Design review of the part shown in the three views and the two pictorial views. Dimensions are in mm from the part's minimum x, y and z. Round coordinates to 2 decimals unless told otherwise and drop trailing zeros. Loops run counter-clockwise (first coordinate to the right, second up) from the corner with the lowest first, then second, coordinate; pieces in that order, holes last. Notation, with made-up numbers: M 86.5,63 L 145.5,63 A23 cw 145.5,98 Z; hole C -7.5,-12 d7. An arc over 180 degrees is marked long. Return JSON: item names as keys, results as strings. Group by question number.
Q1. Clearance check with flat-ended pins moving along their axes: pin 1 Ø4 at (x, y) = (20, 14.5) entering from -Z; pin 2 Ø4 at (y, z) = (9.5, 21.5) entering from -X; pin 3 Ø12 at (x, z) = (25.5, 39.5) entering from -Y; pin 4 Ø6 at (y, z) = (6, 40.5) entering from -X. State where each tip first meets the part, or that it passes through.
Q2. Consider section A-A (z = 5). State the section outline as (x, y) points.
Q3. To check wall thickness, follow line 1 along Z through (x, y) = (25, 17.5); line 2 along Z through (x, y) = (25, 2); line 3 along Y through (x, z) = (12.5, 20). State the ranges of each line that lie inside material, in increasing order.
Q4. Consider section C-C (y = 13.25). State the section outline as (x, z) points.
Q5. Consider section B-B (x = 5). State the section outline as (y, z) points.
Q6. Draft analysis for pull direction Z (two halves, no side actions). For the marked faces 1, 2 and 3, state which applies: pulls with the +Z half, pulls with the -Z half, needs draft (parallel to the pull), parting line crosses it, or undercut.
Q7. Consider section D-D (x = 25). State the section outline as (y, z) points, and give its area (3 significant figures).
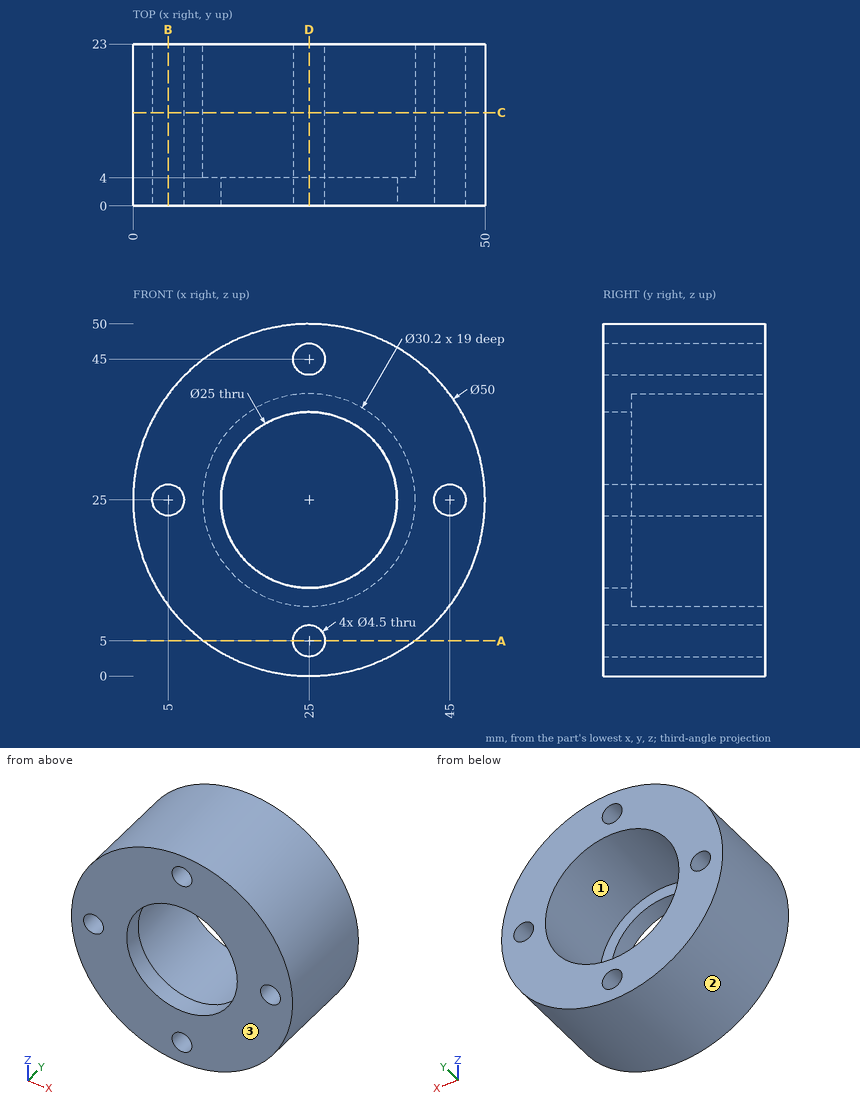
Values:
{
 "1": {"pin 1": "stops at z = 0.18", "pin 2": "stops at x = 0.05", "pin 3": "stops at y = 0", "pin 4": "stops at x = 3.35"},
 "2": {"outline": "M 10,0 L 22.75,0 L 22.75,23 L 10,23 Z; M 27.25,0 L 40,0 L 40,23 L 27.25,23 Z"},
 "3": {"line 1": "z = 0 to 2.75, 7.25 to 9.9, 40.1 to 42.75, 47.25 to 50", "line 2": "z = 0 to 2.75, 7.25 to 12.5, 37.5 to 42.75, 47.25 to 50", "line 3": "y = 0 to 4"},
 "4": {"outline": "C 25,25 d50; hole C 5,25 d4.5; hole C 25,25 d30.2; hole C 25,5 d4.5; hole C 25,45 d4.5; hole C 45,25 d4.5"},
 "5": {"outline": "M 0,10 L 23,10 L 23,22.75 L 0,22.75 Z; M 0,27.25 L 23,27.25 L 23,40 L 0,40 Z"},
 "6": {"face 1": "undercut", "face 2": "parting line crosses it", "face 3": "needs draft"},
 "7": {"outline": "M 0,0 L 23,0 L 23,2.75 L 0,2.75 Z; M 0,7.25 L 23,7.25 L 23,9.9 L 4,9.9 L 4,12.5 L 0,12.5 Z; M 0,37.5 L 4,37.5 L 4,40.1 L 23,40.1 L 23,42.75 L 0,42.75 Z; M 0,47.25 L 23,47.25 L 23,50 L 0,50 Z", "area": "269 mm2"}
}
